Build history of the part. All positions in model axes, mm. A direction names the side the tool comes from. Round coordinates to 2 decimals unless told otherwise and drop trailing zeros. Write each loop counter-clockwise with the first axis right and the second up, starting at its lowest first coordinate (ties: lowest second). Pieces come first, ordered by that corner, then holes. Notation, with made-up numbers: (59, 76) -> (115, 76) arc R26 cw to (115, 104) -> close; hole circle Ø6 at (86.5, 81.5). An arc over 180 degrees is marked (long way). Return JSON: item names as keys, results as strings.
from build123d import *

# Parameters (mm, degrees)
BASE_EXTRUDE_DEPTH      = 193.675
BASE_EXTRUDE_DEPTH_BACK = 193.675
SKETCH2_R               = 8.382
SKETCH2_R_2             = 6.731
HOLES_DEPTH             = 45.45


with BuildPart() as part:
    # Sketch1 → Base-Extrude (new body, two sides)
    with BuildSketch(Plane(origin=(0, 0, 0), x_dir=(0, 0, -1), z_dir=(0, 1, 0))) as base_extrude_sk:
        with BuildLine():
            Line((-73.025, 0), (73.025, 0))
            ThreePointArc((73.025, 0), (84.250320151, -4.649679849), (88.9, -15.875))
            Line((88.9, -15.875), (88.9, -44.45))
            Line((88.9, -44.45), (82.55, -44.45))
            Line((82.55, -44.45), (82.55, -15.875))
            ThreePointArc((82.55, -15.875), (79.760192091, -9.139807909), (73.025, -6.35))
            Line((73.025, -6.35), (-73.025, -6.35))
            ThreePointArc((-73.025, -6.35), (-79.760192091, -9.139807909), (-82.55, -15.875))
            Line((-82.55, -15.875), (-82.55, -44.45))
            Line((-82.55, -44.45), (-88.9, -44.45))
            Line((-88.9, -44.45), (-88.9, -15.875))
            ThreePointArc((-88.9, -15.875), (-84.250320151, -4.649679849), (-73.025, 0))
        make_face()
    extrude(amount=BASE_EXTRUDE_DEPTH)
    extrude(base_extrude_sk.sketch, amount=-BASE_EXTRUDE_DEPTH_BACK)

    # Sketch2 → Holes (cut, through all)
    with BuildSketch(Plane(origin=(0, 0, 0), x_dir=(0, 0, -1), z_dir=(1, 0, 0))):
        with Locations((57.15, 41.275)):
            Circle(SKETCH2_R)
        with Locations((57.15, 104.775)):
            Circle(SKETCH2_R)
        with Locations((57.15, 168.275)):
            Circle(SKETCH2_R)
        with Locations((57.15, -41.275)):
            Circle(SKETCH2_R)
        with Locations((57.15, -104.775)):
            Circle(SKETCH2_R)
        with Locations((57.15, -168.275)):
            Circle(SKETCH2_R)
        with Locations((-57.15, -168.275)):
            Circle(SKETCH2_R)
        with Locations((-57.15, -104.775)):
            Circle(SKETCH2_R)
        with Locations((-57.15, -41.275)):
            Circle(SKETCH2_R)
        with Locations((-57.15, 41.275)):
            Circle(SKETCH2_R)
        with Locations((-57.15, 104.775)):
            Circle(SKETCH2_R)
        with Locations((-57.15, 168.275)):
            Circle(SKETCH2_R)
        with Locations((0, 168.275)):
            Circle(SKETCH2_R_2)
    extrude(amount=HOLES_DEPTH, mode=Mode.SUBTRACT)


solid = part.part
Q1. Saw through at A-A on x = 34. List the corners of the cut face in (y, z) (3 decimals).
Verdict:
{"outline": "(-193.675, -88.9) -> (193.675, -88.9) -> (193.675, -82.55) -> (-193.675, -82.55) -> close; (-193.675, 82.55) -> (193.675, 82.55) -> (193.675, 88.9) -> (-193.675, 88.9) -> close"}
Q2. Saw through at C-C on y = -64. List the corners of the cut face in (x, z) (3 decimals), then the cut area to 3 significant figures.
Verdict:
{"outline": "(0, -73.025) arc R15.875 ccw to (15.875, -88.9) -> (44.45, -88.9) -> (44.45, -82.55) -> (15.875, -82.55) arc R9.525 cw to (6.35, -73.025) -> (6.35, 73.025) arc R9.525 cw to (15.875, 82.55) -> (44.45, 82.55) -> (44.45, 88.9) -> (15.875, 88.9) arc R15.875 ccw to (0, 73.025) -> close", "area": "1,540 mm²"}
Q3. Wall check: L1, parallel to Z at x = 40, y = -15; L2, parallel to Z at x = 3.5, y = 99; L3, parallel to Z at x = 6, y = 163. Give the ranges that are in metal, low to high.
Verdict:
{"L1": "z = -88.9 to -82.55, 82.55 to 88.9", "L2": "z = -82.97 to -63.23, -51.07 to 51.07, 63.23 to 82.97", "L3": "z = -85.45 to -63.66, -50.64 to -4.18, 4.18 to 50.64, 63.66 to 85.45"}
Q4. Two-plate mould, pull along Y, no slides. Class faces 3 (the flat face through (6, -193.675, 0)), 4 (the cylindrical face through (3.131, 41.644, 65.524)), 5 (the flat face through (30, 3, 82.55)): +Y half, -Y half, draft (parallel to the pull), parting line (faces both ways), or undercut.
Verdict:
{"face 3": "-Y half", "face 4": "undercut", "face 5": "draft"}
Q5. Saw through at D-D on z = -1.5. List the corners of the cut face in (x, y) (3 decimals).
Verdict:
{"outline": "(0, -193.675) -> (6.35, -193.675) -> (6.35, 161.713) -> (0, 161.713) -> close; (0, 174.837) -> (6.35, 174.837) -> (6.35, 193.675) -> (0, 193.675) -> close"}
Q6. Pin check, flat tips, straight feed: pin 1 Ø19.5 at (y, z) = (-104.775, 57.15) entering from +X; pin 2 Ø8 at (y, z) = (6.5, 70) entering from +X; pin 3 Ø10 at (y, z) = (147, 57) entering from -X. Stop position of each tip, or through.
Verdict:
{"pin 1": "stops at x = 6.35", "pin 2": "stops at x = 6.4", "pin 3": "stops at x = 0"}
Q7. 3-axis set-ups, long thin cutter, end or side, ignore diameter. For faces 1 (the cylindrical face through (9.21, 2.71, -79.83)), 2 (the cylindrical face through (3.13, -99.11, -50.97)): which of +Z, -Z, +X, -X, +Y, -Y reach the whole face in a straight line?
Verdict:
{"face 1": "+X, +Y, -Y", "face 2": "+X, -X"}
Q8. Saw through at B-B on z = 57.15. List the corners of the cut face in (x, y) (3 decimals), then the cut area to 3 significant figures.
Verdict:
{"outline": "(0, -193.675) -> (6.35, -193.675) -> (6.35, -176.657) -> (0, -176.657) -> close; (0, -159.893) -> (6.35, -159.893) -> (6.35, -113.157) -> (0, -113.157) -> close; (0, -96.393) -> (6.35, -96.393) -> (6.35, -49.657) -> (0, -49.657) -> close; (0, -32.893) -> (6.35, -32.893) -> (6.35, 32.893) -> (0, 32.893) -> close; (0, 49.657) -> (6.35, 49.657) -> (6.35, 96.393) -> (0, 96.393) -> close; (0, 113.157) -> (6.35, 113.157) -> (6.35, 159.893) -> (0, 159.893) -> close; (0, 176.657) -> (6.35, 176.657) -> (6.35, 193.675) -> (0, 193.675) -> close", "area": "1,820 mm²"}
